Here's how the part is built. I have some questions about the finished solid (model axes, mm). A direction names the side the tool comes from. Coordinates: 2 decimals unless noted, no trailing zeros. Write each loop counter-clockwise with the first axis right and the second up, starting at its lowest first coordinate (ties: lowest second). Pieces come first, ordered by that corner, then holes.
Item 1: If we section it at C-C (y = -90): Please give me the cut outline in (x, z).
Item 2: For faces 1 (the face through (150.535, -61.53, -41.38)), 2 (the face through (136, -90, -21.1)), which set-ups out of +Z, -Z, +X, -X, +Y, -Y let a thin tool reach every point of the face, with its end or its side?
Item 3: If we section it at A-A (z = -24.5): Please give me the cut outline in (x, y).
Item 4: We'd pull the mould along Y, two halves only. Please class faces 3 (the face through (136, -103.02, -41)), 4 (the face through (112.806, -75.538, -23.565)), 5 (the face through (120.625, -61.849, -41.38)), 6 (the face through (134, -82, -18.1)): +Y half, -Y half, draft (parallel to the pull), parting line (faces both ways), or undercut.
Item 5: If I drill on line 1 (Z direction, x = 131, y = -56.5); line 2 (Z direction, x = 145, y = -77); line 3 (X direction, y = -63, z = -44), over which ranges is the centre line in solid material (lowest first)?
Item 6: If we section it at B-B (x = 127.5): Please give me the cut outline in (y, z).
Item 7: If we section it at D-D (x = 157): Please give me the cut outline in (y, z).
Item 8: I'm going to push flat-ended pins straight in: pin 1 Ø3.5 at (x, y) = (135.74, -98.57) entering from +Z; pin 2 Ø0.9 at (x, y) = (136.5, -98) entering from +Z; pin 3 Ø6.5 at (x, y) = (141, -80) entering from +Z; pin 4 Ø1 at (y, z) = (-84.5, -50.5) entering from -X. Where does each tip first touch, or does it pass through?
from build123d import *

# Parameters (mm, degrees)
SKETCH018_W             = 42.3
SKETCH018_H             = 42.3
PAD005_DEPTH            = 40
SKETCH019_R             = 11
PAD006_DEPTH            = 3
SKETCH020_R             = 5.1
PAD007_DEPTH            = 21
SKETCH022_R             = 1.5
POCKET011_DEPTH         = 5
CHAMFER001_SIZE         = 5
BODY006_PLACEMENT_ANGLE = 45


with BuildPart() as part:
    # Sketch018 → Pad005 (new body)
    with BuildSketch(Plane.XY):
        Rectangle(SKETCH018_W, SKETCH018_H)
    extrude(amount=PAD005_DEPTH)

    # Sketch019 (on Face6 of Pad005) → Pad006 (join)
    with BuildSketch(Plane.XY.offset(40)):
        Circle(SKETCH019_R)
    extrude(amount=PAD006_DEPTH)

    # Sketch020 (on Face8 of Pad006) → Pad007 (join)
    with BuildSketch(Plane.XY.offset(43)):
        Circle(SKETCH020_R)
    extrude(amount=PAD007_DEPTH)

    # Sketch022 (on Face5 of Pad007) → Pocket011 (cut)
    with BuildSketch(Plane.XY.offset(40)):
        with Locations((-15.5, 15.5)):
            Circle(SKETCH022_R)
        with Locations((15.5, 15.5)):
            Circle(SKETCH022_R)
        with Locations((15.5, -15.5)):
            Circle(SKETCH022_R)
        with Locations((-15.5, -15.5)):
            Circle(SKETCH022_R)
    extrude(amount=-POCKET011_DEPTH, mode=Mode.SUBTRACT)

    # Chamfer001
    chamfer001_edges = [part.edges().sort_by_distance(p)[0] for p in [
        (21.15, 21.15, 20),
        (21.15, -21.15, 20),
        (-21.15, 21.15, 20),
        (-21.15, -21.15, 20),
    ]]
    chamfer(chamfer001_edges, length=CHAMFER001_SIZE)


with BuildPart() as part_1:
    # Body006 placement: moved
    add(part.part.moved(Location((135.7398047638, -76.644724306, -61.1))).rotate(Axis((135.7398047638, -76.644724306, -61.1), (0, 0, -1)), BODY006_PLACEMENT_ANGLE))


solid = part_1.part
Answer list:
1. outline: (119.18, -61.1) - (152.3, -61.1) - (152.3, -21.1) - (119.18, -21.1) - close
2. face 1: +Z, -Z, +X, +Y
2. face 2: +Z
3. outline: (109.36, -80.18) - (132.2, -103.02) - (139.28, -103.02) - (162.11, -80.18) - (162.11, -73.11) - (139.28, -50.27) - (132.2, -50.27) - (109.36, -73.11) - close; hole circle Ø3 at (113.82, -76.64); hole circle Ø3 at (135.74, -98.57); hole circle Ø3 at (135.74, -54.72); hole circle Ø3 at (157.66, -76.64)
4. face 3: -Y half
4. face 4: undercut
4. face 5: +Y half
4. face 6: draft
5. line 1: z = -61.1 to -21.1
5. line 2: z = -61.1 to -18.1
5. line 3: x = 119.47 to 152.01
6. outline: (-98.32, -61.1) - (-54.97, -61.1) - (-54.97, -21.1) - (-69.36, -21.1) - (-69.36, -18.1) - (-83.93, -18.1) - (-83.93, -21.1) - (-98.32, -21.1) - close
7. outline: (-85.3, -61.1) - (-67.99, -61.1) - (-67.99, -21.1) - (-75.3, -21.1) - (-75.3, -26.1) - (-77.99, -26.1) - (-77.99, -21.1) - (-85.3, -21.1) - close
8. pin 1: stops at z = -21.1
8. pin 2: stops at z = -26.1
8. pin 3: stops at z = 2.9
8. pin 4: stops at x = 113.18
